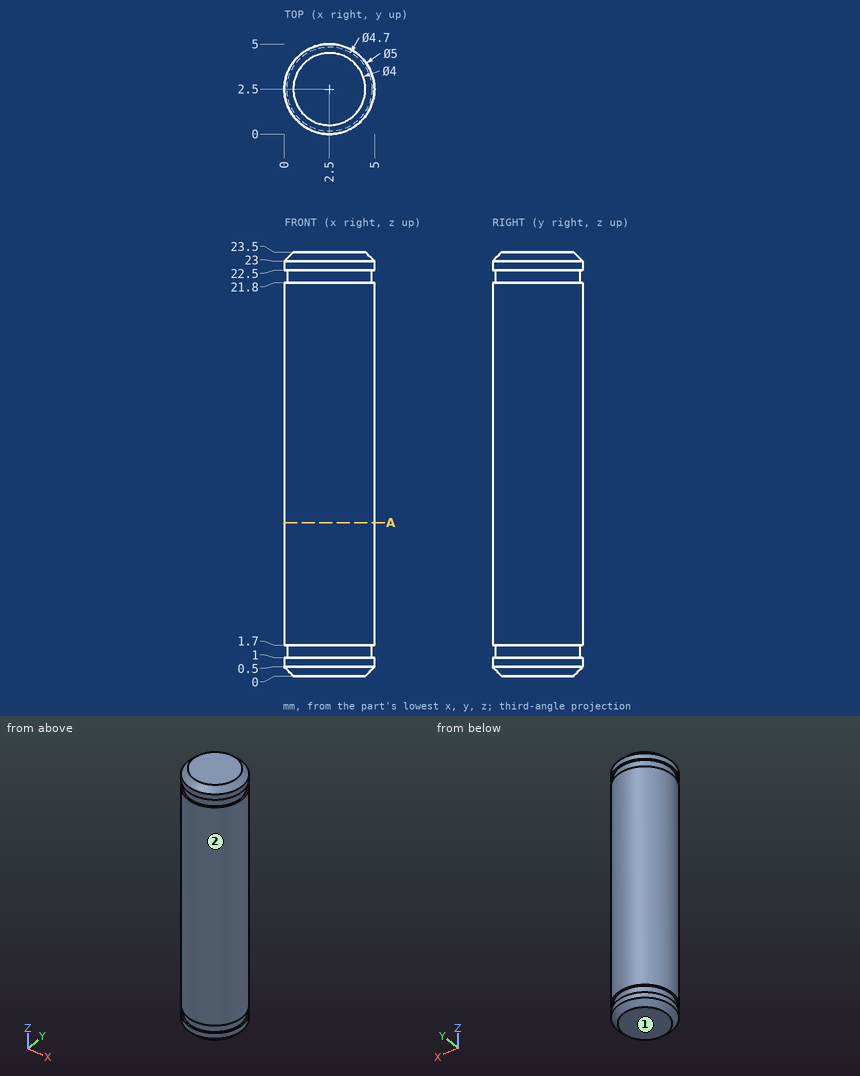
Here's the drawing with two shaded views (mm, measured from the low corner). I have some questions. Coordinates: 2 decimals unless noted, no trailing zeros. Order: outer loops, then holes, each group sorted by start corner. A loop starts at its lowest first (then second) coordinate and runs counter-clockwise, first axis right, second up.
Item 1: I need wall thicknesses on probe 1 along Y at (x, z) = (2.6, 8.75); probe 2 along X at (y, z) = (1.65, 10.75); probe 3 along Y at (x, z) = (0.35, 17.25). Which ranges of each line are inside material? Lowest first, please.
Response values:
probe 1: y = 0 to 5
probe 2: x = 0.15 to 4.85
probe 3: y = 1.22 to 3.78
Item 2: If we section it at A-A, the plane z = 8.5: List the corners of the cut face in (x, y) for me.
Response values:
outline: circle Ø5 at (2.5, 2.5)
Item 3: I'm going to push flat-ended pins straight in: pin 1 Ø1 at (y, z) = (1, 8) entering from +X; pin 2 Ø2.5 at (x, y) = (1.5, 2.5) entering from -Z. Where does each tip first touch, or does it pass through?
Response values:
pin 1: stops at x = 4.79
pin 2: stops at z = 0
Item 4: Thinking about a two-plate mould opening in X: for the marked faces 1 and 2, which applies, pulls with the +X half, pulls with the -X half, needs draft (parallel to the pull), parting line crosses it, or undercut?
Response values:
face 1: needs draft
face 2: parting line crosses it
